Build history of the part. All positions in model axes, mm. A direction names the side the tool comes from. Round coordinates to 2 decimals unless told otherwise and drop trailing zeros. Write each loop counter-clockwise with the first axis right and the second up, starting at its lowest first coordinate (ties: lowest second). Pieces come first, ordered by that corner, then holes. Notation, with made-up numbers: M 59.5,39.5 L 71.5,39.5 A36 ccw 71.5,76.5 Z; hole C 20,-18.75 d9. An arc over 180 degrees is marked long. Write item = value, one per line.
from build123d import *

# Parameters (mm, degrees)
F0_R     = 25.4
F0_R_2   = 21.59
F1_DEPTH = 71.12
F3_DEPTH = 25.4
F4_W     = 13.97
F4_H     = 11.162907
F5_DEPTH = 25.4
F6_W     = 25.4
F6_H     = 71.12
F7_DEPTH = 25.4


with BuildPart() as f1:
    # F0 (on Front) → F1 (new body)
    with BuildSketch(Plane.XZ):
        Circle(F0_R)
        Circle(F0_R_2, mode=Mode.SUBTRACT)
    extrude(amount=F1_DEPTH)

    # F2 (on Top) → F3 (cut)
    with BuildSketch(Plane.XY):
        Polygon((-17.346008, -34.671), (-17.346008, -71.12), (-3.376008, -71.12), (-3.376008, -34.671), (-3.376008, -20.844901), (-25.586616, -20.701003), (-25.596492, -34.671), align=None)
    extrude(amount=-F3_DEPTH, mode=Mode.SUBTRACT)

    # F4 (on Right) → F5 (cut)
    with BuildSketch(Plane.YZ):
        with Locations((-27.686, 5.581453)):
            Rectangle(F4_W, F4_H)
    extrude(amount=-F5_DEPTH, mode=Mode.SUBTRACT)

    # F6 (on Top) → F7 (cut)
    with BuildSketch(Plane.XY):
        with Locations((0, -35.56)):
            Rectangle(F6_W, F6_H)
    extrude(amount=F7_DEPTH, mode=Mode.SUBTRACT)


solid = f1.part
1. Mould opens along Y. For faces 1 (the face through (-22, -34.671, -4)), 2 (the face through (-3.376, -46, -23)), 3 (the face through (6, 0, -21)) say: pulls with the +Y half, pulls with the -Y half, needs draft (parallel to the pull), parting line crosses it, or undercut.
Responses:
face_1 = undercut
face_2 = needs draft
face_3 = pulls with the +Y half
2. Band-saw the part on B-B (z = -12). List the corners of the cut face in (x, y), plus the area to 3 significant figures.
Responses:
outline = M -22.39,-71.12 L -17.95,-71.12 L -17.95,-34.67 L -22.39,-34.67 Z; M -22.39,-20.72 L -17.95,-20.75 L -17.95,0 L -22.39,0 Z; M 17.95,-71.12 L 22.39,-71.12 L 22.39,0 L 17.95,0 Z
area = 570 mm²
3. Flat gauge pins, fed straight in: pin 1 (1.5 mm diameter, centred on x = 15, y = -18, fed in from -Z); pin 2 (2 mm diameter, centred on x = -15, y = -29, fed in from -Z); pin 3 (4 mm diameter, centred on y = -14, z = 11, fed in from +X). Where does each tip first touch, or does it go through?
Responses:
pin_1 = -21.03
pin_2 = 14.5
pin_3 = 23.75
4. Band-saw the part on A-A (y = -30.5). List the corners of the cut face in (x, z).
Responses:
outline = M -22.82,11.16 L -18.48,11.16 A21.59 cw -12.7,17.46 L -12.7,22 A25.4 ccw Z; M -3.38,-25.17 A25.4 ccw 12.7,22 L 12.7,17.46 A21.59 cw -3.38,-21.32 Z
5. Band-saw the part on C-C (x = 16). List the corners of the cut face in (y, z), plus the area to 3 significant figures.
Responses:
outline = M -71.12,-19.73 L 0,-19.73 L 0,-14.5 L -71.12,-14.5 Z; M -71.12,14.5 L 0,14.5 L 0,19.73 L -71.12,19.73 Z
area = 744 mm²
6. Band-saw the part on D-D (z = 4). List the corners of the cut face in (x, y).
Responses:
outline = M -25.08,-71.12 L -21.22,-71.12 L -21.22,-34.67 L -25.08,-34.67 Z; M -25.08,-20.7 L -21.22,-20.7 L -21.22,0 L -25.08,0 Z; M 21.22,-71.12 L 25.08,-71.12 L 25.08,0 L 21.22,0 Z
7. Probe probe 1 along X at (y, z) = (-42.5, 0); probe 2 along Y at (x, z) = (-18.5, -12); probe 3 along Z at (x, y) = (0, -16). List the from-to ranges inside material, lowest first.
Responses:
probe_1 = -25.4 to -21.59, 21.59 to 25.4
probe_2 = -71.12 to -34.67, -20.75 to 0
probe_3 = -25.4 to -21.59
8. Tool access for faces 4 (the face through (13.2, -35.1, -21.7)), 5 (the face through (12.7, -36, 20)), 6 (the face through (-17.346, -53, -16)): list every direction of +Z, -Z, +X, -X, +Y, -Y with a clear straight run to the whole face (end or side of a thin tool).
Responses:
face_4 = +Y, -Y
face_5 = +Z, +Y, -Y
face_6 = -Z, -Y
